```python
from build123d import *

# Parameters (mm, degrees)
SKETCH_1_W               = 60
SKETCH_1_H               = 40
EXTRUDE_1_DEPTH          = 4
CUT_EXTRUDE_1_DEPTH      = 37.276714294
CUT_EXTRUDE_1_DEPTH_BACK = 4
SKETCH_4_R               = 1.5
CUT_EXTRUDE_2_DEPTH      = 10
SKETCH_5_R               = 1.5
CUT_EXTRUDE_3_DEPTH      = 23


with BuildPart() as part:
    # 草图1 → 凸台-拉伸1 (new body)
    with BuildSketch(Plane.XY):
        Rectangle(SKETCH_1_W, SKETCH_1_H)
    extrude(amount=EXTRUDE_1_DEPTH)

    # 草图3 → 切除-拉伸1 (cut, two sides: drawn at the far end of the back side and taken through both)
    with BuildSketch(Plane.XY.offset(4).offset(-CUT_EXTRUDE_1_DEPTH_BACK)):
        Polygon((-30, -14), (-20, 20), (-34.139231405, 23.424173554), (-38.463694215, 14.486950413), (-35.628768595, 5.021181818), (-34.139231405, -14), align=None)
        Polygon((35.628768595, 5.021181818), (34.139231405, -14), (30, -14), (20, 20), (34.139231405, 23.424173554), (38.463694215, 14.486950413), align=None)
    extrude(amount=CUT_EXTRUDE_1_DEPTH + CUT_EXTRUDE_1_DEPTH_BACK, mode=Mode.SUBTRACT)

    # 草图4 → 切除-拉伸2 (cut)
    with BuildSketch(Plane(origin=(0, 0, 0), x_dir=(-1, 0, 0), z_dir=(0, 0, -1))):
        with Locations((22, -17)):
            Circle(SKETCH_4_R)
        with Locations((12, -17)):
            Circle(SKETCH_4_R)
        with Locations((-12, -17)):
            Circle(SKETCH_4_R)
        with Locations((-22, -17)):
            Circle(SKETCH_4_R)
    extrude(amount=-CUT_EXTRUDE_2_DEPTH, mode=Mode.SUBTRACT)

    # 草图5 → 切除-拉伸3 (cut)
    with BuildSketch(Plane.XY.offset(4)):
        with Locations((-11.552312048, -2.99728939)):
            Circle(SKETCH_5_R)
        with Locations((-11.552312048, 9.716256449)):
            Circle(SKETCH_5_R)
        with Locations((8.807786724, -2.99728939)):
            Circle(SKETCH_5_R)
        with Locations((8.807786724, 9.716256449)):
            Circle(SKETCH_5_R)
    extrude(amount=-CUT_EXTRUDE_3_DEPTH, mode=Mode.SUBTRACT)


solid = part.part
```
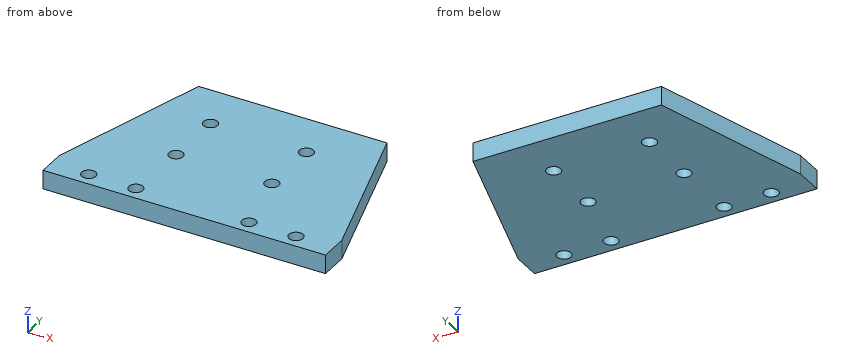
The model under review builds one solid part; all positions refer to its coordinate system, in mm. Give positions to 0.01 mm unless a question says otherwise; leave off trailing zeros. Write each loop counter-clockwise with the first axis right and the second up, starting at its lowest first coordinate (ties: lowest second). Pieces come first, ordered by that corner, then holes. Notation, with made-up numbers: (-14.5, -2.5) - (16.5, -2.5) arc R34 ccw to (16.5, 31.5) - close; hole circle Ø6 at (57.25, 83.5). An arc over 180 degrees is marked (long way). Answer in a Markdown table with one row per item. Add a question column.
1. Wall thickness on line 1 along Y through (x, z) = (-11.5, 0.65); line 2 along X through (y, z) = (10, 1.4); line 3 along Y through (x, z) = (-12, 1.8): over which ranges is each line inside the solid? List them lowest first. Write a range as [from, to].
2. We need section D-D on y = 3. Write out the cut boundary in (x, z), then the cut area to 3 significant figures.
3. Insertion check: P1, Ø1.5, axis at y = 12.5, z = 1.5, coming from the +X side; P2, Ø1.5, axis at y = -6.5, z = 3.5, coming from the -X side; P3, Ø2.5, axis at x = 22, y = -17, coming from the -Z side. Each pin has a flat end and moves straight along its axis. Give the tip position at first contact, or say it passes through.
4. We need section A-A on x = 22. Write out the cut boundary in (y, z).
5. We need section C-C on x = -12. Write out the cut boundary in (y, z), then the cut area to 3 significant figures.
6. We need section B-B on z = 0.65. State how many separate pieces and enclosed holes the cut face has, then the cut area to 3 significant figures.
Ans:
| question | item | result |
|---|---|---|
| 1 | line 1 | y = [-20, -18.41], [-15.59, -4.5], [-1.5, 8.22], [11.22, 20] |
| 1 | line 2 | x = [-22.94, -13.03], [-10.08, 7.33], [10.28, 22.94] |
| 1 | line 3 | y = [-20, -18.5], [-15.5, -4.43], [-1.57, 8.28], [11.15, 20] |
| 2 | outline | (-25, 0) - (25, 0) - (25, 4) - (-25, 4) - close |
| 2 | area | 200 mm^2 |
| 3 | P1 | stops at x = 22.43 |
| 3 | P2 | stops at x = -28.01 |
| 3 | P3 | passes through |
| 4 | outline | (-20, 0) - (-18.5, 0) - (-18.5, 4) - (-20, 4) - close; (-15.5, 0) - (13.2, 0) - (13.2, 4) - (-15.5, 4) - close |
| 5 | outline | (-20, 0) - (-18.5, 0) - (-18.5, 4) - (-20, 4) - close; (-15.5, 0) - (-4.43, 0) - (-4.43, 4) - (-15.5, 4) - close; (-1.57, 0) - (8.28, 0) - (8.28, 4) - (-1.57, 4) - close; (11.15, 0) - (20, 0) - (20, 4) - (11.15, 4) - close |
| 5 | area | 125 mm^2 |
| 6 | separate pieces | 1 |
| 6 | enclosed holes | 8 |
| 6 | area | 2,000 mm^2 |
